Build history of the part. All positions in model axes, mm. Round coordinates to 2 decimals unless told otherwise and drop trailing zeros. Write each loop counter-clockwise with the first axis right and the second up, starting at its lowest first coordinate (ties: lowest second). Pieces come first, ordered by that corner, then holes.
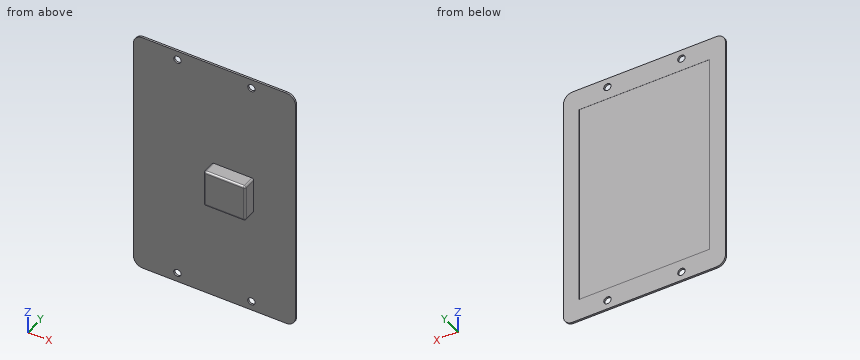
from build123d import *

# Parameters (mm, degrees)
SKETCH_2_W          = 175
SKETCH_2_H          = 270
EXTRUDE_1_DEPTH     = 2
FILLET_1_R          = 10
SKETCH_3_R          = 4
CUT_EXTRUDE_1_DEPTH = 161.888936848
SKETCH_4_W          = 140.906747132
SKETCH_4_H          = 222.417825068
CUT_EXTRUDE_2_DEPTH = 0.1
SKETCH_5_W          = 45
SKETCH_5_H          = 40
EXTRUDE_2_DEPTH     = 15
FILLET_2_R          = 2


with BuildPart() as part:
    # 草图2 → 凸台-拉伸1 (new body)
    with BuildSketch(Plane(origin=(0, 0, 0), x_dir=(1, 0, 0), z_dir=(0, 1, 0))):
        Rectangle(SKETCH_2_W, SKETCH_2_H)
    extrude(amount=EXTRUDE_1_DEPTH)

    # 圆角1
    fillet_1_edges = [part.edges().sort_by_distance(p)[0] for p in [
        (87.5, 1, 135),
        (-87.5, 1, 135),
        (-87.5, 1, -135),
        (87.5, 1, -135),
    ]]
    fillet(fillet_1_edges, radius=FILLET_1_R)

    # 草图3 → 切除-拉伸1 (cut, through all)
    with BuildSketch(Plane(origin=(0, 2, 0), x_dir=(1, 0, 0), z_dir=(0, 1, 0))):
        with Locations(Location((-40, 125, 0), (0, 0, 270))):
            Circle(SKETCH_3_R)
        with Locations(Location((40, 125, 0), (0, 0, 270))):
            Circle(SKETCH_3_R)
        with Locations(Location((40, -125, 0), (0, 0, 270))):
            Circle(SKETCH_3_R)
        with Locations(Location((-40, -125, 0), (0, 0, 270))):
            Circle(SKETCH_3_R)
    extrude(amount=-CUT_EXTRUDE_1_DEPTH, mode=Mode.SUBTRACT)

    # 草图4 → 切除-拉伸2 (cut)
    with BuildSketch(Plane(origin=(0, 2, 0), x_dir=(1, 0, 0), z_dir=(0, 1, 0))):
        Rectangle(SKETCH_4_W, SKETCH_4_H)
    extrude(amount=-CUT_EXTRUDE_2_DEPTH, mode=Mode.SUBTRACT)

    # 草图5 → 凸台-拉伸2 (add)
    with BuildSketch(Plane.XZ):
        with Locations((20, 0)):
            Rectangle(SKETCH_5_W, SKETCH_5_H)
    extrude(amount=EXTRUDE_2_DEPTH)

    # 圆角2
    fillet_2_edges = [part.edges().sort_by_distance(p)[0] for p in [
        (-2.5, -7.5, 20),
        (-2.5, -7.5, -20),
        (42.5, -7.5, -20),
        (42.5, -7.5, 20),
        (-2.5, -15, 0),
        (20, -15, -20),
        (42.5, -15, 0),
        (20, -15, 20),
    ]]
    fillet(fillet_2_edges, radius=FILLET_2_R)


solid = part.part
1) Slice it at A-A (x = -40). Write the cut outline in (y, z).
Results:
outline: (0, -135) - (2, -135) - (2, -129) - (0, -129) - close; (0, -121) - (2, -121) - (2, -111.21) - (1.9, -111.21) - (1.9, 111.21) - (2, 111.21) - (2, 121) - (0, 121) - close; (0, 129) - (2, 129) - (2, 135) - (0, 135) - close
2) Pin check, flat tips, straight feed: pin 1 Ø4 at (y, z) = (-7.5, 0.5) entering from -X; pin 2 Ø6 at (x, z) = (-19.5, -74) entering from -Y; pin 3 Ø5 at (x, z) = (33, -100.5) entering from +Y; pin 4 Ø5 at (x, z) = (40, -125) entering from -Y. Stop position of each tip, or through.
Results:
pin 1: stops at x = -2.5
pin 2: stops at y = 0
pin 3: stops at y = 1.9
pin 4: passes through
3) Slice it at B-B (z = 3). Write the cut outline in (x, y), plus the area to 3 significant figures.
Results:
outline: (-87.5, 0) - (-2.5, 0) - (-2.5, -13) arc R2 ccw to (-0.5, -15) - (40.5, -15) arc R2 ccw to (42.5, -13) - (42.5, 0) - (87.5, 0) - (87.5, 2) - (70.45, 2) - (70.45, 1.9) - (-70.45, 1.9) - (-70.45, 2) - (-87.5, 2) - close
area: 1,010 mm2
4) Slice it at C-C (x = 19). Write the cut outline in (y, z).
Results:
outline: (-15, -18) arc R2 ccw to (-13, -20) - (0, -20) - (0, -135) - (2, -135) - (2, -111.21) - (1.9, -111.21) - (1.9, 111.21) - (2, 111.21) - (2, 135) - (0, 135) - (0, 20) - (-13, 20) arc R2 ccw to (-15, 18) - close
5) Wall check: L1, parallel to X at y = 0.8, z = 125; L2, parallel to X at y = -4.75, z = 13.5; L3, parallel to Y at x = 80, z = 78. Give the ranges that are in metal, low to high.
Results:
L1: x = -87.5 to -44, -36 to 36, 44 to 87.5
L2: x = -2.5 to 42.5
L3: y = 0 to 2
6) Slice it at D-D (y = -7.5). Write the cut outline in (x, z).
Results:
outline: (-2.5, -18) arc R2 ccw to (-0.5, -20) - (40.5, -20) arc R2 ccw to (42.5, -18) - (42.5, 18) arc R2 ccw to (40.5, 20) - (-0.5, 20) arc R2 ccw to (-2.5, 18) - close
